from build123d import *

# Parameters (mm, degrees)
CUT_EXTRUDE1_DEPTH = 33.1
SKETCH3_R          = 10
CUT_EXTRUDE2_DEPTH = 30
CUT_EXTRUDE3_DEPTH = 31.3
SKETCH5_R          = 15
CUT_EXTRUDE4_DEPTH = 8


with BuildPart() as part:
    # Sketch1 → Revolve1 (revolve)
    with BuildSketch(Plane(origin=(0, 0, 0), x_dir=(0, 0, -1), z_dir=(1, 0, 0)), mode=Mode.PRIVATE) as revolve1_sk:
        with BuildLine():
            Line((0, 24.75), (0, 19.9))
            Line((0, 19.9), (11.489270357, 0))
            Line((11.489270357, 0), (66.730344885, 0))
            Line((66.730344885, 0), (77.7, 19))
            Line((77.7, 19), (77.7, 24.2))
            Line((77.7, 24.2), (67.7, 24.2))
            ThreePointArc((67.7, 24.2), (63.4, 22.275), (59.1, 24.2))
            Line((59.1, 24.2), (51.55, 24.2))
            Line((51.55, 24.2), (51, 24.75))
            Line((51, 24.75), (0, 24.75))
        make_face()
    revolve(revolve1_sk.sketch.rotate(Axis((0, 0, 0), (0, 0, 1)), 90), axis=Axis((0, 0, 0), (0, 0, 1)))

    # Sketch2 → Cut-Extrude1 (cut)
    with BuildSketch(Plane.XY):
        with BuildLine():
            Line((-10.420617009, 15.450961894), (-18.591234018, 1.299038106))
            ThreePointArc((-18.591234018, 1.299038106), (-19.341234018, 0), (-18.591234018, -1.299038106))
            Line((-18.591234018, -1.299038106), (-10.420617009, -15.450961894))
            ThreePointArc((-10.420617009, -15.450961894), (-9.670617009, -16.75), (-8.170617009, -16.75))
            Line((-8.170617009, -16.75), (8.170617009, -16.75))
            ThreePointArc((8.170617009, -16.75), (9.670617009, -16.75), (10.420617009, -15.450961894))
            Line((10.420617009, -15.450961894), (18.591234018, -1.299038106))
            ThreePointArc((18.591234018, -1.299038106), (19.341234018, 0), (18.591234018, 1.299038106))
            Line((18.591234018, 1.299038106), (10.420617009, 15.450961894))
            ThreePointArc((10.420617009, 15.450961894), (9.670617009, 16.75), (8.170617009, 16.75))
            Line((8.170617009, 16.75), (-8.170617009, 16.75))
            ThreePointArc((-8.170617009, 16.75), (-9.670617009, 16.75), (-10.420617009, 15.450961894))
        make_face()
    extrude(amount=-CUT_EXTRUDE1_DEPTH, mode=Mode.SUBTRACT)

    # Sketch3 → Cut-Extrude2 (cut)
    with BuildSketch(Plane.XY.offset(-33.1)):
        Circle(SKETCH3_R)
    extrude(amount=-CUT_EXTRUDE2_DEPTH, mode=Mode.SUBTRACT)

    # Sketch4 → Cut-Extrude3 (cut)
    with BuildSketch(Plane(origin=(0, 0, -77.7), x_dir=(-1, 0, 0), z_dir=(0, 0, -1))):
        with BuildLine():
            Line((-12.85, -9.668019485), (-12.85, 9.668019485))
            ThreePointArc((-12.85, 9.668019485), (-12.85, 12.85), (-9.668019485, 12.85))
            Line((-9.668019485, 12.85), (9.668019485, 12.85))
            ThreePointArc((9.668019485, 12.85), (12.85, 12.85), (12.85, 9.668019485))
            Line((12.85, 9.668019485), (12.85, -9.668019485))
            ThreePointArc((12.85, -9.668019485), (12.85, -12.85), (9.668019485, -12.85))
            Line((9.668019485, -12.85), (-9.668019485, -12.85))
            ThreePointArc((-9.668019485, -12.85), (-12.85, -12.85), (-12.85, -9.668019485))
        make_face()
    extrude(amount=-CUT_EXTRUDE3_DEPTH, mode=Mode.SUBTRACT)

    # Sketch5 → Cut-Extrude4 (cut)
    with BuildSketch(Plane.XY.offset(-33.1)):
        Circle(SKETCH5_R)
    extrude(amount=-CUT_EXTRUDE4_DEPTH, mode=Mode.SUBTRACT)


solid = part.part
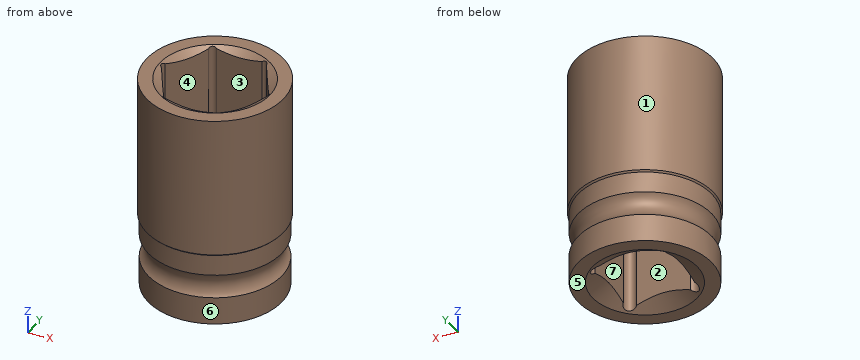
Geometry: final body of the model. Coordinates: model frame, mm. Face numbers are marked on the shaded views. A direction names the side the tool comes from. Give positions to 0.01 mm unless a question says otherwise; leave off trailing zeros. Order: outer loops, then holes, each group sorted by start corner. A loop starts at its lowest first (then second) coordinate and runs counter-clockwise, first axis right, second up. Notation, with made-up numbers: (36, -23.5) -> (53, -23.5) arc R35 ccw to (53, 8.5) -> close; hole circle Ø1 at (33, -12.75). An arc over 180 degrees is marked (long way). Answer as a JSON object with one key per item and string values.
Q1. Draft query along X for the marked faces 4, 5, 6 and 7. Return one class per face: released by +X, released by -X, zero draft, split by the parting line, or undercut.
Entries:
{"face 4": "undercut", "face 5": "zero draft", "face 6": "split by the parting line", "face 7": "undercut"}
Q2. Material intervals for probe 1 along Y at (x, z) = (0, -38); probe 2 along Y at (x, z) = (0, -43.05); probe 3 along X at (y, z) = (-5, -52.5), sorted ascending.
Entries:
{"probe 1": "y = -24.75 to -15, 15 to 24.75", "probe 2": "y = -24.75 to -10, 10 to 24.75", "probe 3": "x = -23.68 to -12.85, 12.85 to 23.68"}
Q3. Access query for the marked faces 1, 2 and 3. Directions: +Z, -Z, +X, -X, +Y, -Y. A direction counts if a zero-diameter tool reaches every point of the face in a straight line with its end or side. Return the directions, or none.
Entries:
{"face 1": "+Z, -Z", "face 2": "-Z", "face 3": "+Z"}
Q4. First-contact query: pin 1 (5 mm diameter, centred on x = 3.5, z = -21, fed in from -Y); pin 2 (23 mm diameter, centred on x = 0, y = 0, fed in from -Z); pin 3 (15 mm diameter, centred on x = 3, y = -0.5, fed in from +Z). Flat tips, straight axial feed; report the tip coordinate or a pass-through.
Entries:
{"pin 1": "stops at y = -24.73", "pin 2": "stops at z = -46.4", "pin 3": "stops at z = -41.1"}
Q5. Section D-D (z = -31.5). Output: boundary loops of the cut face in (x, y), plus the area to 3 significant figures.
Entries:
{"outline": "circle Ø49.5 at (0, 0); hole (-18.59, -1.3) -> (-10.42, -15.45) arc R1.5 ccw to (-8.17, -16.75) -> (8.17, -16.75) arc R1.5 ccw to (10.42, -15.45) -> (18.59, -1.3) arc R1.5 ccw to (18.59, 1.3) -> (10.42, 15.45) arc R1.5 ccw to (8.17, 16.75) -> (-8.17, 16.75) arc R1.5 ccw to (-10.42, 15.45) -> (-18.59, 1.3) arc R1.5 ccw to start", "area": "950 mm^2"}
Q6. Section B-B (z = -53.5). Output: boundary loops of the cut face in (x, y).
Entries:
{"outline": "circle Ø48.4 at (0, 0); hole (-12.85, -9.67) arc R2.25 ccw to (-9.67, -12.85) -> (9.67, -12.85) arc R2.25 ccw to (12.85, -9.67) -> (12.85, 9.67) arc R2.25 ccw to (9.67, 12.85) -> (-9.67, 12.85) arc R2.25 ccw to (-12.85, 9.67) -> close"}
